from build123d import *

# Parameters (mm, degrees)
F0_W         = 25.4
F0_H         = 25.4
F0_W_2       = 20.32
F0_H_2       = 20.32
F1_DEPTH     = 50.8
F2_T1_DEPTH  = 20.32
F2_T3_DEPTH  = 20.32
F2_T9_DEPTH  = 36.6501869736
F2_T15_DEPTH = 36.6501869736
F2_T24_DEPTH = 36.6501869736
F2_T30_DEPTH = 36.6501869736
F2_T39_DEPTH = 36.6501869736
F2_T45_DEPTH = 36.6501869736
F2_T54_DEPTH = 36.6501869736
F2_T60_DEPTH = 36.6501869736


# Not quite as in the source:
# - a fillet or chamfer that OpenCascade refuses, or shapes differently, is made with other operations: its cross-section is extruded or revolved along the edge and cut away or added


with BuildPart() as f1:
    # F0 (on Top) → F1 (new body)
    with BuildSketch(Plane.XY):
        Rectangle(F0_W, F0_H)
        Rectangle(F0_W_2, F0_H_2, mode=Mode.SUBTRACT)
    extrude(amount=F1_DEPTH)

    # F2: chamfer of 6.35 on 4 edges, made by hand

    # F2_s2 → F2_t1 (cut)
    with BuildSketch(Plane.XZ.offset(-10.16)):
        Polygon((-10.16, 44.45), (-16.51, 50.8), (-10.16, 50.8), align=None)
        Polygon((10.16, 44.45), (16.51, 50.8), (10.16, 50.8), align=None)
    extrude(amount=F2_T1_DEPTH, mode=Mode.SUBTRACT)

    # F2_s4 → F2_t3 (cut)
    with BuildSketch(Plane.YZ.offset(-10.16)):
        Polygon((-10.16, 44.45), (-16.51, 50.8), (-10.16, 50.8), align=None)
        Polygon((10.16, 44.45), (16.51, 50.8), (10.16, 50.8), align=None)
    extrude(amount=F2_T3_DEPTH, mode=Mode.SUBTRACT)


with BuildPart() as f2_tool7:
    # F2_s8 → F2_t9 (new body)
    with BuildSketch(Plane.YZ.offset(10.16)):
        Polygon((-10.16, 44.45), (-16.51, 50.8), (-10.16, 50.8), align=None)
    extrude(amount=-F2_T9_DEPTH)

    split(bisect_by=Plane.XZ.offset(12.7), keep=Keep.BOTTOM)

    split(bisect_by=Plane.YZ.offset(-12.7), keep=Keep.TOP)

    split(bisect_by=Plane.YZ.offset(-10.16), keep=Keep.BOTTOM)


with BuildPart() as f2_tool13:
    # F2_s14 → F2_t15 (new body)
    with BuildSketch(Plane.XZ.offset(26.4901869736)):
        Polygon((-10.16, 44.45), (-16.51, 50.8), (-10.16, 50.8), align=None)
    extrude(amount=-F2_T15_DEPTH)

    split(bisect_by=Plane.XZ.offset(12.7), keep=Keep.BOTTOM)

    split(bisect_by=Plane.YZ.offset(-12.7), keep=Keep.TOP)

    split(bisect_by=Plane.XZ.offset(10.16), keep=Keep.TOP)


with BuildPart() as f2_tool7_1:
    add(f2_tool7.part)

    # F2_t19: intersect F2_tool13
    add(f2_tool13.part, mode=Mode.INTERSECT)


with BuildPart() as f1_1:
    add(f1.part)

    # F2_t5: cut F2_tool7
    add(f2_tool7_1.part, mode=Mode.SUBTRACT)


with BuildPart() as f2_tool22:
    # F2_s23 → F2_t24 (new body)
    with BuildSketch(Plane.YZ.offset(-26.4901869736)):
        Polygon((10.16, 44.45), (16.51, 50.8), (10.16, 50.8), align=None)
    extrude(amount=F2_T24_DEPTH)

    split(bisect_by=Plane.XZ.offset(-12.7), keep=Keep.TOP)

    split(bisect_by=Plane.YZ.offset(-12.7), keep=Keep.TOP)

    split(bisect_by=Plane.YZ.offset(-10.16), keep=Keep.BOTTOM)


with BuildPart() as f2_tool28:
    # F2_s29 → F2_t30 (new body)
    with BuildSketch(Plane.XZ.offset(10.16)):
        Polygon((-10.16, 44.45), (-16.51, 50.8), (-10.16, 50.8), align=None)
    extrude(amount=-F2_T30_DEPTH)

    split(bisect_by=Plane.XZ.offset(-12.7), keep=Keep.TOP)

    split(bisect_by=Plane.YZ.offset(-12.7), keep=Keep.TOP)

    split(bisect_by=Plane.XZ.offset(-10.16), keep=Keep.BOTTOM)


with BuildPart() as f2_tool22_1:
    add(f2_tool22.part)

    # F2_t34: intersect F2_tool28
    add(f2_tool28.part, mode=Mode.INTERSECT)


with BuildPart() as f1_2:
    add(f1_1.part)

    # F2_t20: cut F2_tool22
    add(f2_tool22_1.part, mode=Mode.SUBTRACT)


with BuildPart() as f2_tool37:
    # F2_s38 → F2_t39 (new body)
    with BuildSketch(Plane.YZ.offset(-10.16)):
        Polygon((10.16, 44.45), (16.51, 50.8), (10.16, 50.8), align=None)
    extrude(amount=F2_T39_DEPTH)

    split(bisect_by=Plane.YZ.offset(12.7), keep=Keep.BOTTOM)

    split(bisect_by=Plane.XZ.offset(-12.7), keep=Keep.TOP)

    split(bisect_by=Plane.YZ.offset(10.16), keep=Keep.TOP)


with BuildPart() as f2_tool43:
    # F2_s44 → F2_t45 (new body)
    with BuildSketch(Plane.XZ.offset(-26.4901869736)):
        Polygon((10.16, 44.45), (16.51, 50.8), (10.16, 50.8), align=None)
    extrude(amount=F2_T45_DEPTH)

    split(bisect_by=Plane.YZ.offset(12.7), keep=Keep.BOTTOM)

    split(bisect_by=Plane.XZ.offset(-12.7), keep=Keep.TOP)

    split(bisect_by=Plane.XZ.offset(-10.16), keep=Keep.BOTTOM)


with BuildPart() as f2_tool37_1:
    add(f2_tool37.part)

    # F2_t49: intersect F2_tool43
    add(f2_tool43.part, mode=Mode.INTERSECT)


with BuildPart() as f1_3:
    add(f1_2.part)

    # F2_t35: cut F2_tool37
    add(f2_tool37_1.part, mode=Mode.SUBTRACT)


with BuildPart() as f2_tool52:
    # F2_s53 → F2_t54 (new body)
    with BuildSketch(Plane.XZ.offset(-10.16)):
        Polygon((10.16, 44.45), (16.51, 50.8), (10.16, 50.8), align=None)
    extrude(amount=F2_T54_DEPTH)

    split(bisect_by=Plane.XZ.offset(12.7), keep=Keep.BOTTOM)

    split(bisect_by=Plane.YZ.offset(12.7), keep=Keep.BOTTOM)

    split(bisect_by=Plane.XZ.offset(10.16), keep=Keep.TOP)


with BuildPart() as f2_tool58:
    # F2_s59 → F2_t60 (new body)
    with BuildSketch(Plane.YZ.offset(26.4901869736)):
        Polygon((-10.16, 44.45), (-16.51, 50.8), (-10.16, 50.8), align=None)
    extrude(amount=-F2_T60_DEPTH)

    split(bisect_by=Plane.XZ.offset(12.7), keep=Keep.BOTTOM)

    split(bisect_by=Plane.YZ.offset(12.7), keep=Keep.BOTTOM)

    split(bisect_by=Plane.YZ.offset(10.16), keep=Keep.TOP)


with BuildPart() as f2_tool52_1:
    add(f2_tool52.part)

    # F2_t64: intersect F2_tool58
    add(f2_tool58.part, mode=Mode.INTERSECT)


with BuildPart() as f1_4:
    add(f1_3.part)

    # F2_t50: cut F2_tool52
    add(f2_tool52_1.part, mode=Mode.SUBTRACT)


solid = f1_4.part
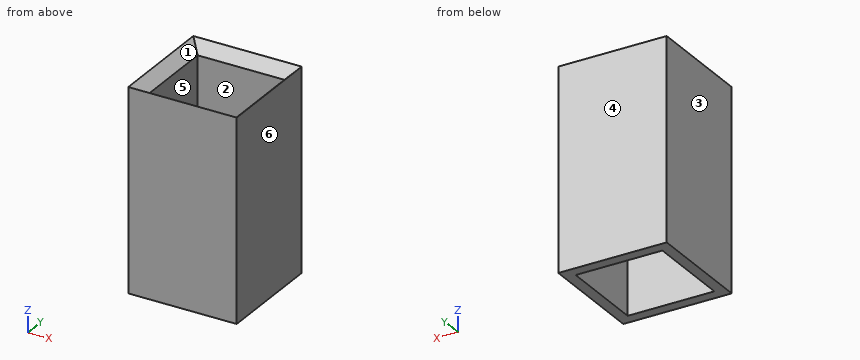
Build history of the part. All positions in model axes, mm. Face numbers are marked on the shaded views. A direction names the side the tool comes from. Coordinates: 2 decimals unless noted, no trailing zeros. Write each loop counter-clockwise with the first axis right and the second up, starting at its lowest first coordinate (ties: lowest second). Pieces come first, ordered by that corner, then holes.
(1) Cut at A-A on y = 6.5. List the corners of the cut face in (x, z), and give its area (3 significant figures).
(2) 3-axis set-ups, long thin cutter, end or side, ignore diameter. For the marked faces 1, 2 and 3: which of +Z, -Z, +X, -X, +Y, -Y reach the whole face in a straight line?
(3) Cut at D-D on y = -11. List the corners of the cut face in (x, z).
(4) Drill centre lines: line 1 (Y direction, x = -1.5, z = 30); line 2 (Z direction, x = 2.25, y = -11.25). Where is each one in solid material? Low to high.
(5) Cut at C-C on z = 10. List the corners of the cut face in (x, y), and give its area (3 significant figures).
(6) Mould opens along X. For the marked faces 4, 5 and 6 say: pulls with the +X half, pulls with the -X half, needs draft (parallel to the pull), parting line crosses it, or undercut.
(7) Pin check, flat tip, straight feed: pin 1 Ø12 at (x, y) = (8, 0) entering from -Z. Stop position of the tip, or through.
Working result:
1. outline: (-12.7, 0) - (-10.16, 0) - (-10.16, 44.45) - (-12.7, 46.99) - close; (10.16, 0) - (12.7, 0) - (12.7, 46.99) - (10.16, 44.45) - close
1. area: 232 mm2
2. face 1: +Z
2. face 2: +Z, -Z
2. face 3: +Z, -Z, -X, +Y, -Y
3. outline: (-12.7, 0) - (12.7, 0) - (12.7, 46.99) - (11, 45.29) - (-11, 45.29) - (-12.7, 46.99) - close
4. line 1: y = -12.7 to -10.16, 10.16 to 12.7
4. line 2: z = 0 to 45.54
5. outline: (-12.7, -12.7) - (12.7, -12.7) - (12.7, 12.7) - (-12.7, 12.7) - close; hole (-10.16, -10.16) - (10.16, -10.16) - (10.16, 10.16) - (-10.16, 10.16) - close
5. area: 232 mm2
6. face 4: needs draft
6. face 5: undercut
6. face 6: pulls with the +X half
7. pin 1: stops at z = 0
